Source: three-view drawing plus pictorial views. Frame: mm from the lowest corner of the part. A direction names the side the tool comes from. Give positions to 0.01 mm unless a question says otherwise; leave off trailing zeros. Loops run counter-clockwise (first coordinate to the right, second up) from the corner with the lowest first, then second, coordinate; pieces in that order, holes last. Notation, with made-up numbers: (27, 28.5) - (70, 28.5) arc R35 ccw to (70, 62.5) - close; hole circle Ø4 at (61, 83.25). An arc over 180 degrees is marked (long way). Put each result on its own line as item: value.
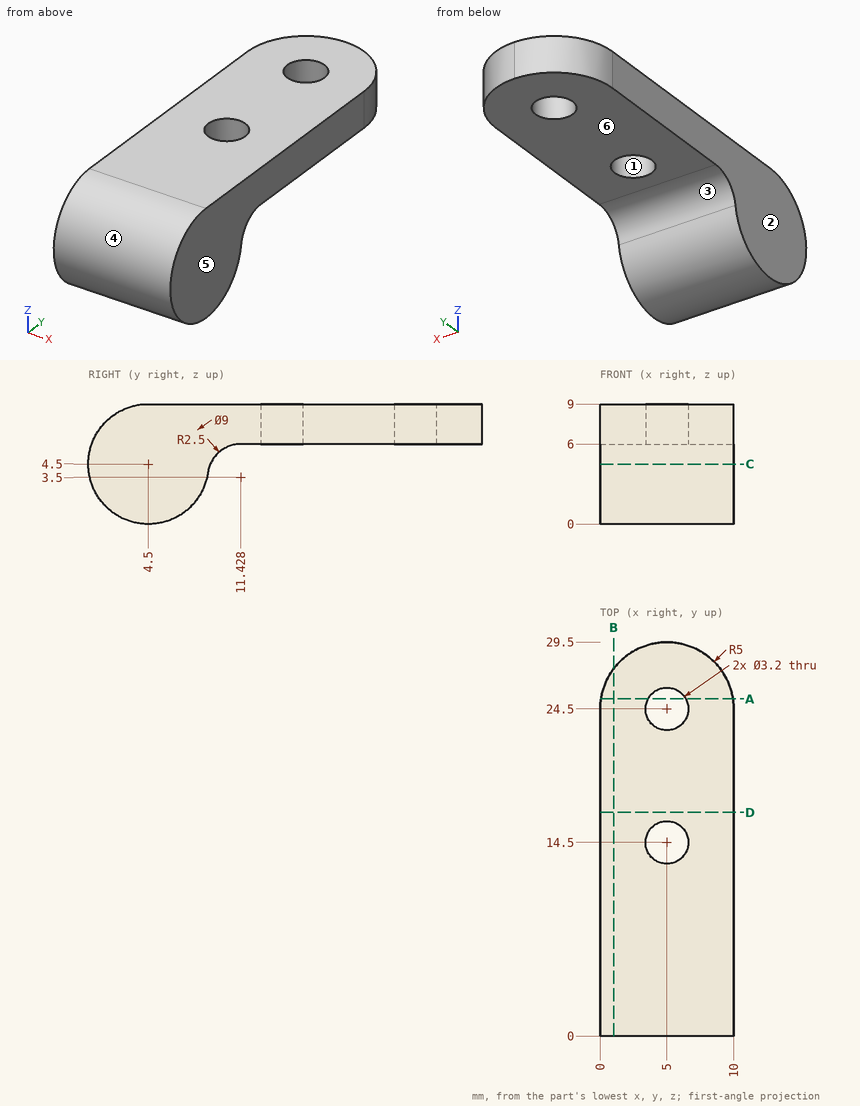
1) Material intervals for line 1 along X through (y, z) = (24.5, 8.25); line 2 along Z through (x, y) = (0.5, 23.25); line 3 along X through (y, z) = (13.25, 7.5), sorted ascending. Write a range as [from, to].
Check result:
line 1: [0, 3.4], [6.6, 10]
line 2: [6, 9]
line 3: [0, 4], [6, 10]
2) Access query for the marked faces 5 and 6. Directions: +Z, -Z, +X, -X, +Y, -Y. A direction counts if a zero-diameter tool reaches every point of the face in a straight line with its end or side. Return the directions, or none.
Check result:
face 5: +Z, -Z, +X, +Y, -Y
face 6: -Z, +X, -X, +Y
3) Section query B-B, the plane x = 1. Output: boundary loops of the cut face in (y, z).
Check result:
outline: (4.5, 9) arc R4.5 ccw (long way) to (8.95, 3.86) arc R2.5 cw to (11.43, 6) - (27.5, 6) - (27.5, 9) - close
4) Section query A-A, the plane y = 25.25. Output: boundary loops of the cut face in (x, z).
Check result:
outline: (0.06, 6) - (3.59, 6) - (3.59, 9) - (0.06, 9) - close; (6.41, 6) - (9.94, 6) - (9.94, 9) - (6.41, 9) - close
5) Section query C-C, the plane z = 4.5. Output: boundary loops of the cut face in (x, y), plus the area to 3 significant figures.
Check result:
outline: (0, 0) - (10, 0) - (10, 9.14) - (0, 9.14) - close
area: 91.4 mm²
6) Mould query, pull axis Y, two halves, no side actions, for the marked faces 1, 2, 3 and 4. Classes: pulls with the +Y half, pulls with the -Y half, needs draft (parallel to the pull), parting line crosses it, or undercut.
Check result:
face 1: undercut
face 2: needs draft
face 3: pulls with the +Y half
face 4: parting line crosses it
7) Pin query (flat end, axial travel): P1, Ø5, axis at x = 5.5, y = 21, coming from the -Z side; P2, Ø5, axis at x = 1.5, z = 5.5, coming from the +Y side; P3, Ø3, axis at x = 5, y = 14.5, coming from the +Z side. Return the tip coordinate at first contact, or that it passes through.
Check result:
P1: z = 6
P2: y = 29.39
P3: through
8) Section query D-D, the plane y = 16.75. Output: boundary loops of the cut face in (x, z).
Check result:
outline: (0, 6) - (10, 6) - (10, 9) - (0, 9) - close
